For this review, take the finished solid that the model builds, in its own axes (mm). Give positions to 0.01 mm unless a question says otherwise; leave off trailing zeros. Order: outer loops, then holes, each group sorted by start corner. A loop starts at its lowest first (then second) coordinate and runs counter-clockwise, first axis right, second up. Notation, with made-up numbers: (-25, -29) - (20, -29) arc R24 ccw to (20, -17) - close; hole circle Ø9 at (54.5, 48.5). An arc over 180 degrees is marked (long way). One line per item, written item: value.
```python
from build123d import *

# Parameters (mm, degrees)
SKETCH_1_W            = 55
SKETCH_1_H            = 32
SKETCH_1_R            = 2.1
EXTRUDE_1_DEPTH       = 10
SKETCH_2_W            = 55
SKETCH_2_H            = 4
EXTRUDE_2_DEPTH       = 10
SKETCH_4_R            = 2.1
SKETCH_4_R_2          = 1.6
EXTRUDE_3_DEPTH       = 10
SKETCH_6_R            = 2.1
EXTRUDE_4_DEPTH       = 10
SKETCH_7_W            = 15
SKETCH_7_H            = 11
CUT_EXTRUDE_1_DEPTH   = 11
EXTRUDE_5_DEPTH       = 10
SKETCH_9_R            = 1.5
CUT_EXTRUDE_2_DEPTH   = 11
SKETCH_10_OUTSIDE_W   = 301.892
SKETCH_10_OUTSIDE_H   = 218.392
SKETCH_10_OUTSIDE_W_2 = 10
SKETCH_10_OUTSIDE_H_2 = 41
CUT_EXTRUDE_3_DEPTH   = 11
FILLET_2_R            = 3


with BuildPart() as part:
    # 草图1 → 凸台-拉伸1 (new body)
    with BuildSketch(Plane(origin=(0, 0, 0), x_dir=(1, 0, 0), z_dir=(0, 1, 0))):
        Rectangle(SKETCH_1_W, SKETCH_1_H)
        with Locations((-12.5, 10)):
            Circle(SKETCH_1_R, mode=Mode.SUBTRACT)
        with Locations((12.5, 10)):
            Circle(SKETCH_1_R, mode=Mode.SUBTRACT)
        with Locations((12.5, -10)):
            Circle(SKETCH_1_R, mode=Mode.SUBTRACT)
        with Locations((-12.5, -10)):
            Circle(SKETCH_1_R, mode=Mode.SUBTRACT)
    extrude(amount=EXTRUDE_1_DEPTH)

    # 草图2 → 凸台-拉伸2 (add)
    with BuildSketch(Plane(origin=(0, 10, 0), x_dir=(1, 0, 0), z_dir=(0, 1, 0))):
        with Locations((0, -18)):
            Rectangle(SKETCH_2_W, SKETCH_2_H)
    extrude(amount=-EXTRUDE_2_DEPTH)

    # 草图4 → 凸台-拉伸3 (add)
    with BuildSketch(Plane(origin=(0, 10, 0), x_dir=(1, 0, 0), z_dir=(0, 1, 0))):
        Polygon((-27.5, -20), (-27.5, -57), (-67.5, -57), (-67.5, -98), (67.5, -98), (67.5, -57), (27.5, -57), (27.5, -20), align=None)
        with Locations((-47.5, -65)):
            Circle(SKETCH_4_R, mode=Mode.SUBTRACT)
        with Locations((-47.5, -90)):
            Circle(SKETCH_4_R, mode=Mode.SUBTRACT)
        with Locations((47.5, -90)):
            Circle(SKETCH_4_R, mode=Mode.SUBTRACT)
        with Locations((47.5, -65)):
            Circle(SKETCH_4_R, mode=Mode.SUBTRACT)
        with Locations((-62, -88)):
            Circle(SKETCH_4_R_2, mode=Mode.SUBTRACT)
        with Locations((-62, -80)):
            Circle(SKETCH_4_R_2, mode=Mode.SUBTRACT)
        with Locations((62, -88)):
            Circle(SKETCH_4_R_2, mode=Mode.SUBTRACT)
        with Locations((62, -80)):
            Circle(SKETCH_4_R_2, mode=Mode.SUBTRACT)
    extrude(amount=-EXTRUDE_3_DEPTH)

    # 草图6 → 凸台-拉伸4 (add)
    with BuildSketch(Plane(origin=(0, 10, 0), x_dir=(1, 0, 0), z_dir=(0, 1, 0))):
        Polygon((-121, -122.5), (-105, -122.5), (-83.215535743, -68), (-67.5, -68), (-67.5, -98), (-89, -142.5), (-121, -142.5), align=None)
        with Locations((-115, -127.5)):
            Circle(SKETCH_6_R, mode=Mode.SUBTRACT)
        with Locations((-95, -127.5)):
            Circle(SKETCH_6_R, mode=Mode.SUBTRACT)
        with Locations((-95, -137.5)):
            Circle(SKETCH_6_R, mode=Mode.SUBTRACT)
        with Locations((-115, -137.5)):
            Circle(SKETCH_6_R, mode=Mode.SUBTRACT)
        Polygon((67.5, -68), (83.215535743, -68), (105, -122.5), (121, -122.5), (121, -142.5), (89, -142.5), (67.5, -98), align=None)
        with Locations((115, -137.5)):
            Circle(SKETCH_6_R, mode=Mode.SUBTRACT)
        with Locations((95, -137.5)):
            Circle(SKETCH_6_R, mode=Mode.SUBTRACT)
        with Locations((95, -127.5)):
            Circle(SKETCH_6_R, mode=Mode.SUBTRACT)
        with Locations((115, -127.5)):
            Circle(SKETCH_6_R, mode=Mode.SUBTRACT)
    extrude(amount=-EXTRUDE_4_DEPTH)

    # 草图7 → 切除-拉伸1 (cut, through all)
    with BuildSketch(Plane(origin=(0, 10, 0), x_dir=(1, 0, 0), z_dir=(0, 1, 0))):
        with Locations((-60, -62.5)):
            Rectangle(SKETCH_7_W, SKETCH_7_H)
        with Locations((60, -62.5)):
            Rectangle(SKETCH_7_W, SKETCH_7_H)
    extrude(amount=-CUT_EXTRUDE_1_DEPTH, mode=Mode.SUBTRACT)

    # 草图8 → 凸台-拉伸5 (add)
    with BuildSketch(Plane(origin=(0, 10, 0), x_dir=(1, 0, 0), z_dir=(0, 1, 0))):
        Polygon((-27.5, -20), (-39.5, -57), (-27.5, -57), align=None)
        Polygon((39.5, -57), (27.5, -57), (27.5, -20), align=None)
    extrude(amount=-EXTRUDE_5_DEPTH)

    # 草图9 → 切除-拉伸2 (cut, through all)
    with BuildSketch(Plane(origin=(0, 10, 0), x_dir=(1, 0, 0), z_dir=(0, 1, 0))):
        with Locations((-30, -67)):
            Circle(SKETCH_9_R)
        with Locations((-15, -67)):
            Circle(SKETCH_9_R)
        with Locations((15, -67)):
            Circle(SKETCH_9_R)
        with Locations((30, -67)):
            Circle(SKETCH_9_R)
    extrude(amount=-CUT_EXTRUDE_2_DEPTH, mode=Mode.SUBTRACT)

    # 草图10 outside → 切除-拉伸3 (cut, through all)
    with BuildSketch(Plane(origin=(0, 10, 0), x_dir=(1, 0, 0), z_dir=(0, 1, 0))):
        with Locations((0, -63.25)):
            Rectangle(SKETCH_10_OUTSIDE_W, SKETCH_10_OUTSIDE_H)
        with Locations((-47.5, -77.5)):
            Rectangle(SKETCH_10_OUTSIDE_W_2, SKETCH_10_OUTSIDE_H_2, mode=Mode.SUBTRACT)
    extrude(amount=-CUT_EXTRUDE_3_DEPTH, mode=Mode.SUBTRACT)

    # 圆角2
    fillet_2_edges = [part.edges().sort_by_distance(p)[0] for p in [
        (-52.5, 5, 57),
        (-42.5, 5, 57),
        (-42.5, 5, 98),
        (-52.5, 5, 98),
    ]]
    fillet(fillet_2_edges, radius=FILLET_2_R)


solid = part.part
```
(1) Take a section at D-D (z = 66). Write out the cut boundary in (x, y), then the cut area to 3 significant figures.
Answers below:
outline: (-52.5, 0) - (-49.35, 0) - (-49.35, 10) - (-52.5, 10) - close; (-45.65, 0) - (-42.5, 0) - (-42.5, 10) - (-45.65, 10) - close
area: 63.1 mm^2
(2) Take a section at B-B (x = -47.5). Write out the cut boundary in (y, z), then the cut area to 3 significant figures.
Answers below:
outline: (0, 57) - (10, 57) - (10, 62.9) - (0, 62.9) - close; (0, 67.1) - (10, 67.1) - (10, 87.9) - (0, 87.9) - close; (0, 92.1) - (10, 92.1) - (10, 98) - (0, 98) - close
area: 326 mm^2
(3) For P1, Ø1, axis at x = -50.5, y = 6.5, coming from the -Z side, flat-tipped, find the tip position at first contact; note if it passes through.
Answers below:
P1: stops at z = 57.04
(4) Take a section at A-A (z = 90). Write out the cut boundary in (x, y), then the cut area to 3 significant figures.
Answers below:
outline: (-52.5, 0) - (-49.6, 0) - (-49.6, 10) - (-52.5, 10) - close; (-45.4, 0) - (-42.5, 0) - (-42.5, 10) - (-45.4, 10) - close
area: 58.0 mm^2
(5) Draft analysis for pull direction Z (two halves, no side actions). For faces 1 (the face through (-43.36, 4.93, 97.1)), 2 (the face through (-45.56, 5.07, 90.8)), 3 (the face through (-48, 0, 77)), state which applies: pulls with the +Z half, pulls with the -Z half, needs draft (parallel to the pull), parting line crosses it, or undercut.
Answers below:
face 1: pulls with the +Z half
face 2: undercut
face 3: needs draft
(6) Take a section at C-C (y = 3.5). Write out the cut boundary in (x, z), then the cut area to 3 significant figures.
Answers below:
outline: (-52.5, 60) arc R3 ccw to (-49.5, 57) - (-45.5, 57) arc R3 ccw to (-42.5, 60) - (-42.5, 95) arc R3 ccw to (-45.5, 98) - (-49.5, 98) arc R3 ccw to (-52.5, 95) - close; hole circle Ø4.2 at (-47.5, 65); hole circle Ø4.2 at (-47.5, 90)
area: 375 mm^2
(7) Wall thickness on line 1 (Z direction, x = -47.5, y = 9.25); line 2 (X direction, y = 3.5, z = 65); line 3 (Z direction, x = -48, y = 0.75): over which ranges is each line inside the solid? List them lowest first. Write a range as from..to.
Answers below:
line 1: z = 57..62.9, 67.1..87.9, 92.1..98
line 2: x = -52.5..-49.6, -45.4..-42.5
line 3: z = 57..62.96, 67.04..87.96, 92.04..98
